from build123d import *

# Parameters (mm, degrees)
BOSS_EXTRUDE1_DEPTH = 175


with BuildPart() as part:
    # Model → Boss-Extrude1 (new body)
    with BuildSketch(Plane.XY):
        with BuildLine():
            Line((-3, 8.3), (-3, 9.7))
            ThreePointArc((-3, 9.7), (-3.087867966, 9.912132034), (-3.3, 10))
            Line((-3.3, 10), (-9, 10))
            ThreePointArc((-9, 10), (-9.707106781, 9.707106781), (-10, 9))
            Line((-10, 9), (-10, 3.3))
            ThreePointArc((-10, 3.3), (-9.912132034, 3.087867966), (-9.7, 3))
            Line((-9.7, 3), (-8.3, 3))
            ThreePointArc((-8.3, 3), (-8.087867966, 3.087867966), (-8, 3.3))
            Line((-8, 3.3), (-8, 6))
            Line((-8, 6), (-7.060660172, 6))
            Line((-7.060660172, 6), (-4, 2.939339828))
            Line((-4, 2.939339828), (-4, 0.653589838))
            ThreePointArc((-4, 0.653589838), (-3.982962913, 0.524180316), (-3.933012702, 0.403589838))
            Line((-3.933012702, 0.403589838), (-3.7, 0))
            Line((-3.7, 0), (-3.933012702, -0.403589838))
            ThreePointArc((-3.933012702, -0.403589838), (-3.982962913, -0.524180316), (-4, -0.653589838))
            Line((-4, -0.653589838), (-4, -2.939339828))
            Line((-4, -2.939339828), (-7.060660172, -6))
            Line((-7.060660172, -6), (-8, -6))
            Line((-8, -6), (-8, -3.3))
            ThreePointArc((-8, -3.3), (-8.087867966, -3.087867966), (-8.3, -3))
            Line((-8.3, -3), (-9.7, -3))
            ThreePointArc((-9.7, -3), (-9.912132034, -3.087867966), (-10, -3.3))
            Line((-10, -3.3), (-10, -9))
            ThreePointArc((-10, -9), (-9.707106781, -9.707106781), (-9, -10))
            Line((-9, -10), (-3.3, -10))
            ThreePointArc((-3.3, -10), (-3.087867966, -9.912132034), (-3, -9.7))
            Line((-3, -9.7), (-3, -8.3))
            ThreePointArc((-3, -8.3), (-3.087867966, -8.087867966), (-3.3, -8))
            Line((-3.3, -8), (-6, -8))
            Line((-6, -8), (-6, -7.060660172))
            Line((-6, -7.060660172), (-2.939339828, -4))
            Line((-2.939339828, -4), (-0.653589838, -4))
            ThreePointArc((-0.653589838, -4), (-0.524180316, -3.982962913), (-0.403589838, -3.933012702))
            Line((-0.403589838, -3.933012702), (0, -3.7))
            Line((0, -3.7), (0.403589838, -3.933012702))
            ThreePointArc((0.403589838, -3.933012702), (0.524180316, -3.982962913), (0.653589838, -4))
            Line((0.653589838, -4), (2.939339828, -4))
            Line((2.939339828, -4), (6, -7.060660172))
            Line((6, -7.060660172), (6, -8))
            Line((6, -8), (3.3, -8))
            ThreePointArc((3.3, -8), (3.087867966, -8.087867966), (3, -8.3))
            Line((3, -8.3), (3, -9.7))
            ThreePointArc((3, -9.7), (3.087867966, -9.912132034), (3.3, -10))
            Line((3.3, -10), (9, -10))
            ThreePointArc((9, -10), (9.707106781, -9.707106781), (10, -9))
            Line((10, -9), (10, -3.3))
            ThreePointArc((10, -3.3), (9.912132034, -3.087867966), (9.7, -3))
            Line((9.7, -3), (8.3, -3))
            ThreePointArc((8.3, -3), (8.087867966, -3.087867966), (8, -3.3))
            Line((8, -3.3), (8, -6))
            Line((8, -6), (7.060660172, -6))
            Line((7.060660172, -6), (4, -2.939339828))
            Line((4, -2.939339828), (4, -0.653589838))
            ThreePointArc((4, -0.653589838), (3.982962913, -0.524180316), (3.933012702, -0.403589838))
            Line((3.933012702, -0.403589838), (3.7, 0))
            Line((3.7, 0), (3.933012702, 0.403589838))
            ThreePointArc((3.933012702, 0.403589838), (3.982962913, 0.524180316), (4, 0.653589838))
            Line((4, 0.653589838), (4, 2.939339828))
            Line((4, 2.939339828), (7.060660172, 6))
            Line((7.060660172, 6), (8, 6))
            Line((8, 6), (8, 3.3))
            ThreePointArc((8, 3.3), (8.087867966, 3.087867966), (8.3, 3))
            Line((8.3, 3), (9.7, 3))
            ThreePointArc((9.7, 3), (9.912132034, 3.087867966), (10, 3.3))
            Line((10, 3.3), (10, 9))
            ThreePointArc((10, 9), (9.707106781, 9.707106781), (9, 10))
            Line((9, 10), (3.3, 10))
            ThreePointArc((3.3, 10), (3.087867966, 9.912132034), (3, 9.7))
            Line((3, 9.7), (3, 8.3))
            ThreePointArc((3, 8.3), (3.087867966, 8.087867966), (3.3, 8))
            Line((3.3, 8), (6, 8))
            Line((6, 8), (6, 7.060660172))
            Line((6, 7.060660172), (2.939339828, 4))
            Line((2.939339828, 4), (0.653589838, 4))
            ThreePointArc((0.653589838, 4), (0.524180316, 3.982962913), (0.403589838, 3.933012702))
            Line((0.403589838, 3.933012702), (0, 3.7))
            Line((0, 3.7), (-0.403589838, 3.933012702))
            ThreePointArc((-0.403589838, 3.933012702), (-0.524180316, 3.982962913), (-0.653589838, 4))
            Line((-0.653589838, 4), (-2.939339828, 4))
            Line((-2.939339828, 4), (-6, 7.060660172))
            Line((-6, 7.060660172), (-6, 8))
            Line((-6, 8), (-3.3, 8))
            ThreePointArc((-3.3, 8), (-3.087867966, 8.087867966), (-3, 8.3))
        make_face()
        with BuildLine():
            ThreePointArc((-2.1, 0), (-1.48492424, -1.48492424), (0, -2.1))
            ThreePointArc((0, -2.1), (1.48492424, -1.48492424), (2.1, 0))
            ThreePointArc((2.1, 0), (1.48492424, 1.48492424), (0, 2.1))
            ThreePointArc((0, 2.1), (-1.48492424, 1.48492424), (-2.1, 0))
        make_face(mode=Mode.SUBTRACT)
    extrude(amount=BOSS_EXTRUDE1_DEPTH)


solid = part.part
Geometry check sheet. Reference: the model listing, model coordinates, mm. A direction names the side the tool comes from. Give positions to 0.01 mm unless a question says otherwise; leave off trailing zeros.
(1) Thickness scan on L1, parallel to X at y = 4.5, z = 24; L2, parallel to Y at x = 5.25, z = 36; L3, parallel to X at y = -5.5, z = 90.5. Record the ranges inside material, lowest first.
From the geometry:
L1: x = -10 to -8, -5.56 to -3.44, 3.44 to 5.56, 8 to 10
L2: y = -10 to -8, -6.31 to -4.19, 4.19 to 6.31, 8 to 10
L3: x = -10 to -8, -6.56 to -4.44, 4.44 to 6.56, 8 to 10
(2) Set-up check for faces 5 (the flat face through (-6, -10, 86)), 6 (the flat face through (-5.55, 4.49, 86.28)): record each of +Z, -Z, +X, -X, +Y, -Y from which the full face is reachable in a straight line by a thin tool's end or side.
From the geometry:
face 5: +Z, -Z, +X, -X, -Y
face 6: +Z, -Z
(3) Depth check by flat-ended pin: pin 1 Ø1.1 at (y, z) = (2, 60.5) entering from +X; pin 2 Ø1.8 at (y, z) = (-2, 90) entering from -X; pin 3 Ø0.7 at (x, z) = (-2, 107) entering from -Y; pin 4 Ø1.5 at (x, y) = (2, 6) entering from +Z. Enter the tip coordinate at first touch or a pass-through.
From the geometry:
pin 1: stops at x = 4
pin 2: stops at x = -4
pin 3: stops at y = -4
pin 4: passes through
(4) Release check for a two-part mould opening along Y. For faces 1 (the flat face through (6, 10, 86)), 2 (the flat face through (-0.1, 2.4, 0)), 3 (the flat face through (6, -10, 86)), 4 (the flat face through (-8, -5, 86)) record: released by +Y, released by -Y, zero draft, split by the parting line, or undercut.
From the geometry:
face 1: released by +Y
face 2: zero draft
face 3: released by -Y
face 4: undercut
